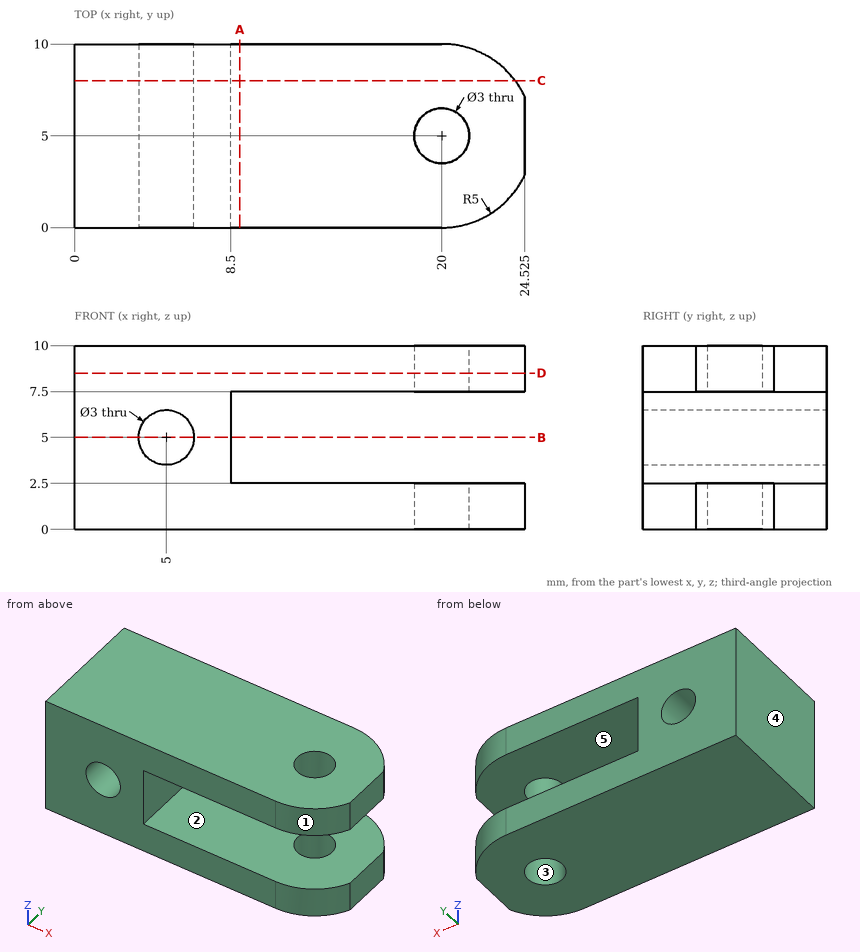
Geometry check sheet. Reference: drawing and pictorial views, mm from the part's lowest x, y, z. A direction names the side the tool comes from. Round coordinates to 2 decimals unless told otherwise and drop trailing zeros. Loops run counter-clockwise (first coordinate to the right, second up) from the corner with the lowest first, then second, coordinate; pieces in that order, holes last.
1. Sectioned sample at D-D on z = 8.5. Record the boundary of the cut face in (x, y) (3 decimals), and give its area (3 significant figures).
2. Scan lines: probe 1 along Y at (x, z) = (20, 1.65); probe 2 along Z at (x, y) = (9.25, 9.5); probe 3 along X at (y, z) = (5, 1.45) (3 decimals). Record each from-to range of solid material in increasing order.
3. Set-up check for the marked faces 4 and 5: record each of +Z, -Z, +X, -X, +Y, -Y from which the full face is reachable in a straight line by a thin tool's end or side.
4. Sectioned sample at A-A on x = 9. Record the boundary of the cut face in (y, z), and give its area (3 significant figures).
5. Mould release check, pull along Y, two halves, no side actions. Record for the marked faces 1, 2 and 3: released by +Y, released by -Y, zero draft, split by the parting line, or undercut.
6. Gauge pin test, flat end, axial feed: pin 1 Ø5.5 at (y, z) = (6.5, 5.5) entering from +X (3 decimals). Record the tip position at first contact, or that the pin passes through.
7. Sectioned sample at B-B on z = 5. Record the boundary of the cut face in (x, y), and give its area (3 significant figures).
8. Sectioned sample at C-C on y = 8. Record the boundary of the cut face in (x, z).
Recorded:
1. outline: (0, 0) - (20, 0) arc R5 ccw to (24.525, 2.873) - (24.525, 7.127) arc R5 ccw to (20, 10) - (0, 10) - close; hole circle Ø3 at (20, 5)
1. area: 231 mm2
2. probe 1: y = 0 to 3.5, 6.5 to 10
2. probe 2: z = 0 to 2.5, 7.5 to 10
2. probe 3: x = 0 to 18.5, 21.5 to 24.525
3. face 4: +Z, -Z, -X, +Y, -Y
3. face 5: +X, +Y, -Y
4. outline: (0, 0) - (10, 0) - (10, 2.5) - (0, 2.5) - close; (0, 7.5) - (10, 7.5) - (10, 10) - (0, 10) - close
4. area: 50.0 mm2
5. face 1: released by -Y
5. face 2: zero draft
5. face 3: undercut
6. pin 1: stops at x = 24.525
7. outline: (0, 0) - (3.5, 0) - (3.5, 10) - (0, 10) - close; (6.5, 0) - (8.5, 0) - (8.5, 10) - (6.5, 10) - close
7. area: 55.0 mm2
8. outline: (0, 0) - (24, 0) - (24, 2.5) - (8.5, 2.5) - (8.5, 7.5) - (24, 7.5) - (24, 10) - (0, 10) - close; hole circle Ø3 at (5, 5)
